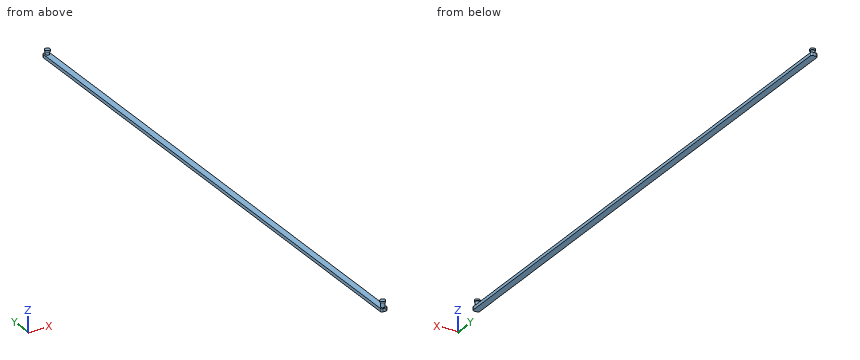
Autodesk Inventor part; units mm, degrees
ref_plane "YZ Plane" through (0, 0, 0) normal (1, 0, 0) x (0, 1, 0)
ref_plane "XZ Plane" through (0, 0, 0) normal (0, 1, 0) x (-1, 0, 0)
ref_plane "XY Plane" through (0, 0, 0) normal (0, 0, 1) x (1, 0, 0)
sketch "Skizze1" plane through (0, 0, 0) normal (0, 0, 1) x (1, 0, 0)
  line L0 (-15, 1712.029) -> (-5, 1712.029)
  line L1 (0, 1707.029) -> (0, 5)
  line L2 (-5, 0) -> (-15, 0)
  line L3 (-20, 5) -> (-20, 1707.029)
  circle A0 centre (-10, 10) radius 5.95
  circle A1 centre (-10, 1702.029) radius 5.95
  arc A2 (-15, 1712.029) -> (-20, 1707.029) centre (-15, 1707.029) ccw
  arc A3 (0, 1707.029) -> (-5, 1712.029) centre (-5, 1707.029) ccw
  arc A4 (-20, 5) -> (-15, 0) centre (-15, 5) ccw
  arc A5 (-5, 0) -> (0, 5) centre (-5, 5) ccw
  point P0 (0, 0)
  point P1 (-20, 1712.029)
  point P2 (0, 1712.029)
  dimension "d0" = 20
  dimension "d2" = 11.9
  dimension "d3" = 10
  dimension "d4" = 10
  dimension "d5" = 11.9
  dimension "d6" = 10
  dimension "d7" = 1692.029
  dimension "d8" = 10
  dimension "d9" = 5
extrude "Extrusion1" add sketch "Skizze1" against normal blind 10 contours L0 A3 L1 A5 L2 A4 L3 A2 | A0 | A1
extrude "Extrusion2" add sketch "Skizze1" along normal blind 10 contours A1
sketch "Skizze2" plane through (-10, 1702.029, 10) normal (0, 0, 1) x (1, 0, 0)
  circle A0 centre (0, 0) radius 8
  point P0 (10, -1702.029)
  dimension "d14" = 16
extrude "Extrusion3" add sketch "Skizze2" along normal blind 5
extrude "Extrusion4" add sketch "Skizze1" along normal blind 15 contours A0
sketch "Skizze3" plane through (-10, 10, 15) normal (0, 0, 1) x (1, 0, 0)
  circle A0 centre (0, 0) radius 8
  point P0 (10, -10)
  dimension "d19" = 16
extrude "Extrusion5" add sketch "Skizze3" along normal blind 5
properties part number "Lenkung_verbindung"
Geometry: final body of the model. Coordinates: model frame, mm. Round coordinates to 2 decimals unless told otherwise and drop trailing zeros. Order: outer loops, then holes, each group sorted by start corner. A loop starts at its lowest first (then second) coordinate and runs counter-clockwise, first axis right, second up. Notation, with made-up numbers: M 42.5,26 L 48.5,26 A15 cw 48.5,55 Z; hole C 47.25,87.5 d1. An arc over 180 degrees is marked long. One line per item, written item: value.
(1) Cut plane A-A (x = -10). Return the cut outline in (y, z), and give its area (3 significant figures).
Result sheet:
outline: M 0,-10 L 1712.03,-10 L 1712.03,0 L 1707.98,0 L 1707.98,10 L 1710.03,10 L 1710.03,15 L 1694.03,15 L 1694.03,10 L 1696.08,10 L 1696.08,0 L 15.95,0 L 15.95,15 L 18,15 L 18,20 L 2,20 L 2,15 L 4.05,15 L 4.05,0 L 0,0 Z
area: 17,600 mm2
(2) Cut plane B-B (y = 787). Return the cut outline in (x, z), and give its area (3 significant figures).
Result sheet:
outline: M -20,-10 L 0,-10 L 0,0 L -20,0 Z
area: 200 mm2
(3) Pin query (flat end, axial travel): P1, Ø2, axis at x = -6, z = 4.5, coming from the -Y side; P2, Ø8, axis at x = -2.5, y = 277.5, coming from the +Z side; P3, Ø12, axis at x = -15, z = 14.5, coming from the -Y side. Return the tip coordinate at first contact, or that it passes through.
Result sheet:
P1: y = 4.86
P2: z = 0
P3: y = 2
(4) Line query: probe 1 along Y at (x, z) = (-11, 8.25); probe 2 along Z at (x, y) = (-11, 1428.5); probe 3 along Y at (x, z) = (-4.5, 17.5). Output: solid intervals per line, ascending. Write a range as [from, to].
Result sheet:
probe 1: [4.13, 15.87], [1696.16, 1707.89]
probe 2: [-10, 0]
probe 3: [4.19, 15.81]
